Verification items for the finished model (mm, model axes). A direction names the side the tool comes from. Coordinates: 2 decimals unless noted, no trailing zeros. Order: outer loops, then holes, each group sorted by start corner. A loop starts at its lowest first (then second) coordinate and runs counter-clockwise, first axis right, second up. Notation, with made-up numbers: (-22, 49) -> (-4, 49) arc R13 cw to (-4, 70) -> close; hole circle Ø2 at (-14.75, 62). An arc over 180 degrees is marked (long way). Answer as CSV lines item,"result".
```python
from build123d import *

# Parameters (mm, degrees)
F0_R     = 1.397
F1_DEPTH = 6.35
F2_W     = 35.56
F2_H     = 63.5
F3_DEPTH = 3.81
F4_W     = 35.56
F4_H     = 50.8
F5_DEPTH = 25.4


with BuildPart() as f1:
    # F0 (on Top) → F1 (new body)
    with BuildSketch(Plane.XY):
        with BuildLine():
            ThreePointArc((-22.352, 0), (-20.955, -1.397), (-19.558, 0))
            ThreePointArc((-19.558, 0), (-20.955, 1.397), (-22.352, 0))
        make_face()
        Polygon((-24.13, 31.75), (-24.13, 0), (-24.13, -31.75), (-17.78, -31.75), (17.78, -31.75), (24.13, -31.75), (24.13, 31.75), (17.78, 31.75), (-17.78, 31.75), align=None)
        with Locations((-20.955, -25.4)):
            Circle(F0_R, mode=Mode.SUBTRACT)
        with Locations((-20.955, -19.05)):
            Circle(F0_R, mode=Mode.SUBTRACT)
        with Locations((-20.955, -12.7)):
            Circle(F0_R, mode=Mode.SUBTRACT)
        with Locations((-20.955, -6.35)):
            Circle(F0_R, mode=Mode.SUBTRACT)
        with Locations((20.955, -25.4)):
            Circle(F0_R, mode=Mode.SUBTRACT)
        with Locations((20.955, -19.05)):
            Circle(F0_R, mode=Mode.SUBTRACT)
        with Locations((20.955, -12.7)):
            Circle(F0_R, mode=Mode.SUBTRACT)
        with Locations((20.955, -6.35)):
            Circle(F0_R, mode=Mode.SUBTRACT)
        with BuildLine():
            ThreePointArc((-22.352, 0), (-20.955, 1.397), (-19.558, 0))
            ThreePointArc((-19.558, 0), (-20.955, -1.397), (-22.352, 0))
        make_face(mode=Mode.SUBTRACT)
        with Locations((-20.955, 6.35)):
            Circle(F0_R, mode=Mode.SUBTRACT)
        with Locations((-20.955, 12.7)):
            Circle(F0_R, mode=Mode.SUBTRACT)
        with Locations((-20.955, 19.05)):
            Circle(F0_R, mode=Mode.SUBTRACT)
        with Locations((-20.955, 25.4)):
            Circle(F0_R, mode=Mode.SUBTRACT)
        with Locations((20.955, 0)):
            Circle(F0_R, mode=Mode.SUBTRACT)
        with Locations((20.955, 6.35)):
            Circle(F0_R, mode=Mode.SUBTRACT)
        with Locations((20.955, 12.7)):
            Circle(F0_R, mode=Mode.SUBTRACT)
        with Locations((20.955, 19.05)):
            Circle(F0_R, mode=Mode.SUBTRACT)
        with Locations((20.955, 25.4)):
            Circle(F0_R, mode=Mode.SUBTRACT)
    extrude(amount=F1_DEPTH)

    # F2 (on face) → F3 (cut)
    with BuildSketch(Plane.XY.offset(6.35)):
        Rectangle(F2_W, F2_H)
    extrude(amount=-F3_DEPTH, mode=Mode.SUBTRACT)

    # F4 (on face) → F5 (cut)
    with BuildSketch(Plane.XY.offset(2.54)):
        Rectangle(F4_W, F4_H)
    extrude(amount=-F5_DEPTH, mode=Mode.SUBTRACT)


solid = f1.part
```
Item 1: Thickness scan on line 1 (X direction, y = -25.5, z = 0.75); line 2 (X direction, y = 23, z = 4.75); line 3 (X direction, y = 20, z = 5.5). Record the ranges inside material, lowest first.
Answer list:
line 1,"-24.13 to -22.35, -19.56 to 19.56, 22.35 to 24.13"
line 2,"-24.13 to -17.78, 17.78 to 24.13"
line 3,"-24.13 to -21.98, -19.93 to -17.78, 17.78 to 19.93, 21.98 to 24.13"
Item 2: Tool access check on faces 5 (the flat face through (0, 29, 2.54)), 6 (the flat face through (0, -25.4, 1)), 7 (the flat face through (-17.78, 0, 3)), 8 (the flat face through (-23, 0, 6.35)). Record the directions out of +Z, -Z, +X, -X, +Y, -Y that give a thin tool (end or side, any length) a straight path to the whole face; none if there is none.
Answer list:
face 5,"+Z, +Y, -Y"
face 6,"+Z, -Z"
face 7,"+Z"
face 8,"+Z, +X, -X, +Y, -Y"
Item 3: Section check A-A, the plane x = 0. Record the boundary of the cut face in (y, z).
Answer list:
outline,"(-31.75, 0) -> (-25.4, 0) -> (-25.4, 2.54) -> (-31.75, 2.54) -> close; (25.4, 0) -> (31.75, 0) -> (31.75, 2.54) -> (25.4, 2.54) -> close"
Item 4: Section check B-B, the plane z = 4.75. Count the separate pieces of the cut face and the enclosed holes in it, plus the area to 3 significant figures.
Answer list:
separate pieces,"2"
enclosed holes,"18"
area,"696 mm2"
Item 5: Section check D-D, the plane y = 19.05. Record the boundary of the cut face in (x, z).
Answer list:
outline,"(-24.13, 0) -> (-22.35, 0) -> (-22.35, 6.35) -> (-24.13, 6.35) -> close; (-19.56, 0) -> (-17.78, 0) -> (-17.78, 6.35) -> (-19.56, 6.35) -> close; (17.78, 0) -> (19.56, 0) -> (19.56, 6.35) -> (17.78, 6.35) -> close; (22.35, 0) -> (24.13, 0) -> (24.13, 6.35) -> (22.35, 6.35) -> close"
Item 6: Depth check by flat-ended pin: pin 1 Ø3 at (x, y) = (-0.5, 28) entering from +Z. Enter the tip coordinate at first touch or a pass-through.
Answer list:
pin 1,"z = 2.54"
Item 7: Release check for a two-part mould opening along Y. For faces 1 (the flat face through (19, 0, 6.35)), 2 (the cylindrical face through (-22.35, -6.29, 3.13)), 3 (the flat face through (0, -31.75, 2)), 4 (the flat face through (0, 31.75, 2)) record: +Y half, -Y half, draft (parallel to the pull), parting line (faces both ways), or undercut.
Answer list:
face 1,"draft"
face 2,"undercut"
face 3,"-Y half"
face 4,"+Y half"
Item 8: Section check C-C, the plane y = -22.5. Record the boundary of the cut face in (x, z), plus the area to 3 significant figures.
Answer list:
outline,"(-24.13, 0) -> (-17.78, 0) -> (-17.78, 6.35) -> (-24.13, 6.35) -> close; (17.78, 0) -> (24.13, 0) -> (24.13, 6.35) -> (17.78, 6.35) -> close"
area,"80.6 mm2"
